Check sheet for the modelled part. Datum: model origin and axes. Units: mm. Face numbers are marked on the shaded views. Round coordinates to 2 decimals unless told otherwise and drop trailing zeros. Order: outer loops, then holes, each group sorted by start corner. A loop starts at its lowest first (then second) coordinate and runs counter-clockwise, first axis right, second up.
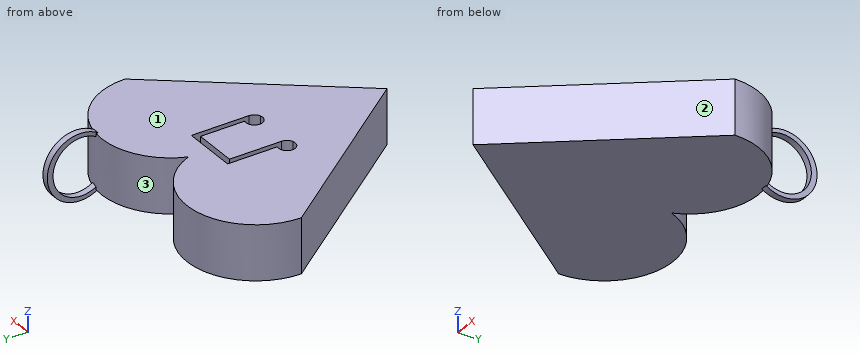
from build123d import *

# Parameters (mm, degrees)
F1_DEPTH = 6.35
F3_DEPTH = 1.905
F7_DEPTH = 0.381
F8_DEPTH = 0.381


with BuildPart() as f1:
    # F0 (on Top) → F1 (new body)
    with BuildSketch(Plane.XY):
        with BuildLine():
            Line((-15.4625402968, 20.1511748434), (0, 0))
            Line((0, 0), (15.4625402968, 20.1511748434))
            ThreePointArc((15.4625402968, 20.1511748434), (8.9216538352, 28.0088478457), (0, 23.0158213526))
            ThreePointArc((0, 23.0158213526), (-8.9175015723, 27.9864351215), (-15.4625402968, 20.1511748434))
        make_face()
    extrude(amount=F1_DEPTH)

    # F2 (on face) → F3 (cut)
    with BuildSketch(Plane.XY.offset(6.35)):
        with BuildLine():
            Line((2.54, 13.0019117156), (2.54, 14.7979629398))
            ThreePointArc((2.54, 14.7979629398), (1.27, 13.8999373277), (2.54, 13.0019117156))
        make_face()
        with BuildLine():
            ThreePointArc((2.54, 13.0019117156), (3.0002129933, 13.3500111963), (3.175, 13.8999373277))
            ThreePointArc((3.175, 13.8999373277), (3.0002129933, 14.4498634591), (2.54, 14.7979629398))
            Line((2.54, 14.7979629398), (2.54, 13.0019117156))
        make_face()
        with BuildLine():
            Line((3.175, 13.8999373277), (3.175, 19.9324373277))
            Line((3.175, 19.9324373277), (2.54, 19.9324373277))
            Line((2.54, 19.9324373277), (2.54, 14.7979629398))
            ThreePointArc((2.54, 14.7979629398), (3.0002129933, 14.4498634591), (3.175, 13.8999373277))
        make_face()
        Polygon((3.175, 20.5674373277), (-3.175, 20.5674373277), (-3.175, 19.9324373277), (-2.54, 19.9324373277), (2.54, 19.9324373277), (3.175, 19.9324373277), align=None)
        with BuildLine():
            Line((-2.54, 19.9324373277), (-3.175, 19.9324373277))
            Line((-3.175, 19.9324373277), (-3.175, 14.7979629398))
            ThreePointArc((-3.175, 14.7979629398), (-2.7147870067, 14.4498634591), (-2.54, 13.8999373277))
            Line((-2.54, 13.8999373277), (-2.54, 19.9324373277))
        make_face()
        with BuildLine():
            ThreePointArc((-2.54, 13.8999373277), (-2.7147870067, 14.4498634591), (-3.175, 14.7979629398))
            Line((-3.175, 14.7979629398), (-3.175, 13.0019117156))
            ThreePointArc((-3.175, 13.0019117156), (-2.7147870067, 13.3500111963), (-2.54, 13.8999373277))
        make_face()
        with BuildLine():
            Line((-3.175, 13.0019117156), (-3.175, 14.7979629398))
            ThreePointArc((-3.175, 14.7979629398), (-4.445, 13.8999373277), (-3.175, 13.0019117156))
        make_face()
    extrude(amount=-F3_DEPTH, mode=Mode.SUBTRACT)

    # F6 (on offset) → F7 (join)
    with BuildSketch(Plane.YZ.offset(8.9154)):
        with BuildLine():
            ThreePointArc((27.804363519, 0), (33.7204202608, 3.175), (27.804363519, 6.35))
            Line((27.804363519, 6.35), (27.804363519, 5.842))
            ThreePointArc((27.804363519, 5.842), (33.0560059571, 3.175), (27.804363519, 0.508))
            Line((27.804363519, 0.508), (27.804363519, 0))
        make_face()
    extrude(amount=F7_DEPTH)

    # F6 (on offset) → F8 (join)
    with BuildSketch(Plane.YZ.offset(8.9154)):
        with BuildLine():
            ThreePointArc((27.804363519, 0), (33.7204202608, 3.175), (27.804363519, 6.35))
            Line((27.804363519, 6.35), (27.804363519, 5.842))
            ThreePointArc((27.804363519, 5.842), (33.0560059571, 3.175), (27.804363519, 0.508))
            Line((27.804363519, 0.508), (27.804363519, 0))
        make_face()
    extrude(amount=-F8_DEPTH)


solid = f1.part
1) Sectioned sample at B-B on z = 1.5. Record the cut outline in (x, y).
2) Sectioned sample at A-A on z = 5.25. Record the cut outline in (x, y) (1 decimal).
3) Gauge pin test, flat ends, axial feed: pin 1 (1 mm diameter, centred on x = 7.5, z = 3, fed in from -Y); pin 2 (1 mm diameter, centred on x = -1, z = 5, fed in from -Y); pin 3 (1 mm diameter, centred on y = 11, z = 5, fed in from -X). Record the tip position at first contact, or that the pin passes through.
4) Sectioned sample at C-C on y = 16. Record the cut outline in (x, z) (3 decimals).
5) Scan lines: line 1 (Z direction, x = -5, y = 9); line 2 (X direction, y = 15, z = 6.25) (3 decimals); line 3 (X direction, y = 24.5, z = 3.5). Record each from-to range of solid material in increasing order.
6) Sectioned sample at D-D on x = -7. Record the cut outline in (y, z).
7) Draft check along X on the marked faces 1, 2 and 3. Enter one of: pulls with the +X half, pulls with the -X half, needs draft (parallel to the pull), parting line crosses it, or undercut.
Values found:
1. outline: (-15.46, 20.15) - (0, 0) - (15.46, 20.15) arc R8 ccw to (0, 23.02) arc R8 ccw to start; (8.53, 32.6) - (9.3, 32.6) - (9.3, 33.33) - (8.53, 33.33) - close
2. outline: (-15.5, 20.2) - (0, 0) - (15.5, 20.2) arc R8 ccw to (0, 23) arc R8 ccw to start; (8.5, 32.3) - (9.3, 32.3) - (9.3, 33.1) - (8.5, 33.1) - close; hole (-3.2, 14.8) arc R1 ccw (long way) to (-2.5, 13.9) - (-2.5, 19.9) - (2.5, 19.9) - (2.5, 14.8) arc R1 ccw (long way) to (3.2, 13.9) - (3.2, 20.6) - (-3.2, 20.6) - close
3. pin 1: stops at y = 9.12
3. pin 2: stops at y = 0.65
3. pin 3: stops at x = -8.82
4. outline: (-12.277, 0) - (12.277, 0) - (12.277, 6.35) - (3.175, 6.35) - (3.175, 4.445) - (2.54, 4.445) - (2.54, 6.35) - (-2.54, 6.35) - (-2.54, 4.445) - (-3.175, 4.445) - (-3.175, 6.35) - (-12.277, 6.35) - close
5. line 1: z = 0 to 6.35
5. line 2: x = -11.51 to -3.175, -2.54 to 2.54, 3.175 to 11.51
5. line 3: x = -14.16 to -0.76, 0.76 to 14.17
6. outline: (9.12, 0) - (28.11, 0) - (28.11, 6.35) - (9.12, 6.35) - close
7. face 1: needs draft
7. face 2: pulls with the +X half
7. face 3: undercut
